Geometry: final body of the model. Coordinates: model frame, mm. A direction names the side the tool comes from. Give positions to 0.01 mm unless a question says otherwise; leave off trailing zeros. Loops run counter-clockwise (first coordinate to the right, second up) from the corner with the lowest first, then second, coordinate; pieces in that order, holes last. Notation, with made-up numbers: (-22, -10) - (-11, -10) arc R26 cw to (-11, 16) - close; hole circle Ø6 at (4.25, -12.5). An arc over 180 degrees is marked (long way). Use one line per item in the form item = value.
```python
from build123d import *

# Parameters (mm, degrees)
SKETCH1_W           = 90
SKETCH1_H           = 75
BOSS_EXTRUDE1_DEPTH = 5
SKETCH2_R           = 1.5
CUT_EXTRUDE1_DEPTH  = 5
SKETCH3_R           = 4.5
CUT_EXTRUDE2_DEPTH  = 2
FILLET1_R           = 3


with BuildPart() as part:
    # Sketch1 → Boss-Extrude1 (new body)
    with BuildSketch(Plane(origin=(0, 0, 0), x_dir=(1, 0, 0), z_dir=(0, 1, 0))):
        Rectangle(SKETCH1_W, SKETCH1_H)
    extrude(amount=BOSS_EXTRUDE1_DEPTH)

    # Sketch2 → Cut-Extrude1 (cut)
    with BuildSketch(Plane(origin=(0, 5, 0), x_dir=(1, 0, 0), z_dir=(0, 1, 0))):
        with Locations(Location((-39.37, 27.94, 0), (0, 0, 270))):
            Circle(SKETCH2_R)
        with Locations(Location((39.37, 27.94, 0), (0, 0, 270))):
            Circle(SKETCH2_R)
        with Locations(Location((39.37, -27.94, 0), (0, 0, 270))):
            Circle(SKETCH2_R)
        with Locations(Location((-39.37, -27.94, 0), (0, 0, 270))):
            Circle(SKETCH2_R)
    extrude(amount=-CUT_EXTRUDE1_DEPTH, mode=Mode.SUBTRACT)

    # Sketch3 → Cut-Extrude2 (cut)
    with BuildSketch(Plane.XZ):
        with Locations(Location((-22.5, -32.5, 0), (0, 0, 270))):
            Circle(SKETCH3_R)
        with Locations(Location((-22.5, 32.5, 0), (0, 0, 270))):
            Circle(SKETCH3_R)
        with Locations(Location((22.5, 32.5, 0), (0, 0, 270))):
            Circle(SKETCH3_R)
        with Locations(Location((22.5, -32.5, 0), (0, 0, 270))):
            Circle(SKETCH3_R)
    extrude(amount=-CUT_EXTRUDE2_DEPTH, mode=Mode.SUBTRACT)

    # Fillet1
    fillet1_edges = [part.edges().sort_by_distance(p)[0] for p in [
        (45, 2.5, 37.5),
        (-45, 2.5, 37.5),
        (-45, 2.5, -37.5),
        (45, 2.5, -37.5),
    ]]
    fillet(fillet1_edges, radius=FILLET1_R)


solid = part.part
```
(1) Access query for faces 1 (the face through (44.1, 2.54, 36.64)), 2 (the face through (23, 2, 33)). Directions: +Z, -Z, +X, -X, +Y, -Y. A direction counts if a zero-diameter tool reaches every point of the face in a straight line with its end or side. Return the directions, or none.
Solution:
face_1 = +Z, +X, +Y, -Y
face_2 = -Y
(2) Pull-direction query (Z, two-part tool) for faces 3 (the face through (-44.14, 2.54, -36.6)), 4 (the face through (-1, 2, 37.5)), 5 (the face through (23, 2, -32)); classes: released by +Z, released by -Z, zero draft, split by the parting line, or undercut.
Solution:
face_3 = released by -Z
face_4 = released by +Z
face_5 = undercut
(3) Material intervals for L1, parallel to X at y = 2.05, z = 27.94; L2, parallel to X at y = 0.75, z = -32.5, sorted ascending. Write a range as from..to.
Solution:
L1 = -45..-40.87, -37.87..37.87, 40.87..45
L2 = -45..-27, -18..18, 27..45
(4) Cut plane B-B (z = -32.5). Return the cut outline in (x, y), plus the area to 3 significant figures.
Solution:
outline = (-45, 0) - (-27, 0) - (-27, 2) - (-18, 2) - (-18, 0) - (18, 0) - (18, 2) - (27, 2) - (27, 0) - (45, 0) - (45, 5) - (-45, 5) - close
area = 414 mm2
(5) Pin query (flat end, axial travel): P1, Ø2.5, axis at x = 20.5, z = 30.5, coming from the -Y side. Return the tip coordinate at first contact, or that it passes through.
Solution:
P1 = 2
(6) Cut plane A-A (x = -39.37). Return the cut outline in (y, z).
Solution:
outline = (0, -37.5) - (5, -37.5) - (5, -29.44) - (0, -29.44) - close; (0, -26.44) - (5, -26.44) - (5, 26.44) - (0, 26.44) - close; (0, 29.44) - (5, 29.44) - (5, 37.5) - (0, 37.5) - close
